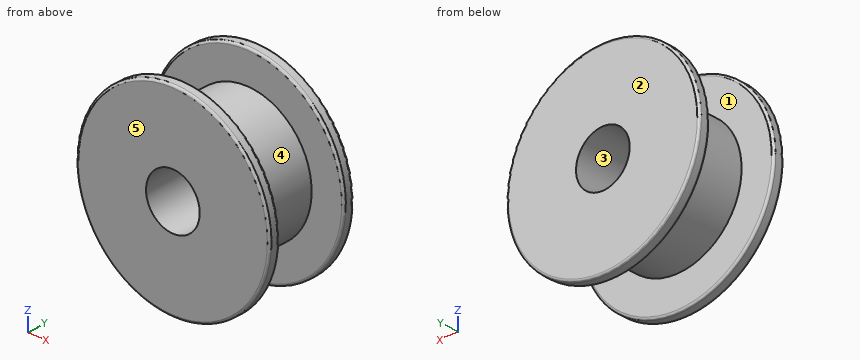
from build123d import *

# Parameters (mm, degrees)
SKETCH1_R           = 9
BOSS_EXTRUDE1_DEPTH = 1
SKETCH2_R           = 6
BOSS_EXTRUDE2_DEPTH = 6.5
SKETCH3_R           = 9
BOSS_EXTRUDE3_DEPTH = 1
SKETCH4_R           = 2.5
CUT_EXTRUDE1_DEPTH  = 16.305227865
FILLET1_R           = 0.2


with BuildPart() as part:
    # Sketch1 → Boss-Extrude1 (new body)
    with BuildSketch(Plane(origin=(0, 0, 0), x_dir=(1, 0, 0), z_dir=(0, 1, 0))):
        with Locations(Location((0, 0, 0), (0, 0, 270))):
            Circle(SKETCH1_R)
    extrude(amount=BOSS_EXTRUDE1_DEPTH)

    # Sketch2 → Boss-Extrude2 (add)
    with BuildSketch(Plane(origin=(0, 1, 0), x_dir=(1, 0, 0), z_dir=(0, 1, 0))):
        with Locations(Location((0, 0, 0), (0, 0, 90))):
            Circle(SKETCH2_R)
    extrude(amount=BOSS_EXTRUDE2_DEPTH)

    # Sketch3 → Boss-Extrude3 (add)
    with BuildSketch(Plane(origin=(0, 7.5, 0), x_dir=(1, 0, 0), z_dir=(0, 1, 0))):
        with Locations(Location((0, 0, 0), (0, 0, 270))):
            Circle(SKETCH3_R)
    extrude(amount=BOSS_EXTRUDE3_DEPTH)

    # Sketch4 → Cut-Extrude1 (cut, through all)
    with BuildSketch(Plane(origin=(0, 8.5, 0), x_dir=(1, 0, 0), z_dir=(0, 1, 0))):
        with Locations(Location((0, 0, 0), (0, 0, 270))):
            Circle(SKETCH4_R)
    extrude(amount=-CUT_EXTRUDE1_DEPTH, mode=Mode.SUBTRACT)

    # Fillet1
    fillet1_edges = [part.edges().sort_by_distance(p)[0] for p in [
        (0, 8.5, -9),
        (0, 0, -9),
        (0, 1, -9),
        (0, 7.5, -9),
    ]]
    fillet(fillet1_edges, radius=FILLET1_R)


solid = part.part
The listing builds one solid part. Answer for the finished solid, in the listing's coordinates (mm). Face numbers are marked on the shaded views. A direction names the side the tool comes from. Round coordinates to 2 decimals unless told otherwise and drop trailing zeros. Write each loop counter-clockwise with the first axis right and the second up, starting at its lowest first coordinate (ties: lowest second). Pieces come first, ordered by that corner, then holes. Notation, with made-up numbers: M 45.5,-25.75 L 55.5,-25.75 A33 cw 55.5,7.25 Z; hole C 5.5,-18.75 d6. An arc over 180 degrees is marked long. Write each question's results on one line, items separated by ' | '. Start each with the question number.
(1) For the marked faces 1 and 2, determine the directions among +Z, -Z, +X, -X, +Y, -Y from which every point of the face is accessible in a straight line to the end or side of a thin tool.
(2) The part is cut by section A-A, the plane x = 0. Write down the section's boundary in (y, z), and give its area (3 significant figures).
(3) Find the intervals of material crossed by line 1 (Y direction, x = -6.5, z = 0.25); line 2 (X direction, y = 3, z = 0); line 3 (Z direction, x = -3.75, y = 5.5), in increasing order.
(4) The part is cut by section B-B, the plane z = 0. Write down the section's boundary in (x, y).
(5) Determine the mould class of the marked faces 3, 4 and 5 for opening direction X: +X half, -X half, draft (parallel to the pull), parting line (faces both ways), or undercut.
(6) The part is cut by section C-C, the plane y = 1.5. Write down the section's boundary in (x, z), and give its area (3 significant figures).
(7) Each of these flat-tipped pins is pushed along its axis until it touches: P1, Ø4.5, axis at x = 0, z = 0, coming from the +Y side; P2, Ø5, axis at y = 1, z = -6, coming from the -X side; P3, Ø1.5, axis at x = 2, y = 6.5, coming from the +Z side. Where does it stop, or does it pass through?
Worked answers:
1) face 1: none | face 2: +Z, -Z, +X, -X, +Y
2) outline: M 0,-8.8 A0.2 ccw 0.2,-9 L 0.8,-9 A0.2 ccw 1,-8.8 L 1,-6 L 7.5,-6 L 7.5,-8.8 A0.2 ccw 7.7,-9 L 8.3,-9 A0.2 ccw 8.5,-8.8 L 8.5,-2.5 L 0,-2.5 Z; M 0,2.5 L 8.5,2.5 L 8.5,8.8 A0.2 ccw 8.3,9 L 7.7,9 A0.2 ccw 7.5,8.8 L 7.5,6 L 1,6 L 1,8.8 A0.2 ccw 0.8,9 L 0.2,9 A0.2 ccw 0,8.8 Z | area: 71.4 mm²
3) line 1: y = 0 to 1, 7.5 to 8.5 | line 2: x = -6 to -2.5, 2.5 to 6 | line 3: z = -4.68 to 4.68
4) outline: M -9,0.2 A0.2 ccw -8.8,0 L -2.5,0 L -2.5,8.5 L -8.8,8.5 A0.2 ccw -9,8.3 L -9,7.7 A0.2 ccw -8.8,7.5 L -6,7.5 L -6,1 L -8.8,1 A0.2 ccw -9,0.8 Z; M 2.5,0 L 8.8,0 A0.2 ccw 9,0.2 L 9,0.8 A0.2 ccw 8.8,1 L 6,1 L 6,7.5 L 8.8,7.5 A0.2 ccw 9,7.7 L 9,8.3 A0.2 ccw 8.8,8.5 L 2.5,8.5 Z
5) face 3: undercut | face 4: parting line | face 5: draft
6) outline: C 0,0 d12; hole C 0,0 d5 | area: 93.5 mm²
7) P1: passes through | P2: stops at x = -8.29 | P3: stops at z = 5.87
